Can you work these out from the model? Positions are in its coordinate system, mm. Face numbers are marked on the shaded views. A direction names the side the tool comes from. Round coordinates to 2 decimals unless told otherwise and drop trailing zeros. Write each loop counter-clockwise with the first axis right and the second up, starting at its lowest first coordinate (ties: lowest second). Pieces come first, ordered by that corner, then holes.
Q1. Please list where these lines run through material, in increasing order: line 1 along X through (y, z) = (-50, -14.5); line 2 along X through (y, z) = (-43, -4.5); line 3 along Z through (x, y) = (-13.5, -34).
Q2. We'd pull the mould along Z, two halves only. Please class the marked faces 6, 7 and 8: +Z half, -Z half, draft (parallel to the pull), parting line (faces both ways), or undercut.
Q3. If we section it at B-B (z = 0): Please give me the cut outline in (x, y), plus the area to 3 significant figures.
Q4. For the marked faces 1, 2, 3, 4 and 5, which set-ups out of +Z, -Z, +X, -X, +Y, -Y let a thin tool reach every point of the face, with its end or its side?
Q5. If we section it at A-A (y = -25.5): Please give me the cut outline in (x, z), plus the area to 3 significant figures.
Q6. If we section it at C-C (y = -11): Please give me the cut outline in (x, z), plus the area to 3 significant figures.
Q7. I'm going to push flat-ended pins straight in: pin 1 Ø21 at (x, z) = (-61, 31) entering from -Y; pin 2 Ø8 at (y, z) = (-27, 13.5) entering from -X; pin 3 Ø21 at (x, y) = (-61.5, -27.5) entering from +Z; pin 4 Ø3 at (x, z) = (21, -3.5) entering from +Y. Where does each tip first touch, or does it pass through?
Q8. If we section it at D-D (x = -25): Please give me the cut outline in (y, z).
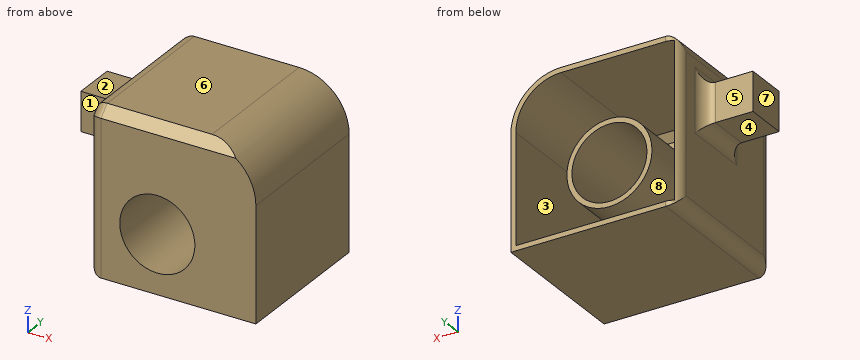
from build123d import *

# Parameters (mm, degrees)
F0_W          = 84.9268175662
F0_H          = 83.4368709475
F1_DEPTH      = 76.2
F2_SIZE       = 5.08
F3_R          = 25.4
F5_D          = 38.1
F8_T          = -2.54
F9_W          = 21.4254707098
F9_H          = 19.7638887912
F10_DEPTH     = 25.4
F11_T1_DEPTH  = 19.7638887912
F11_T3_DEPTH  = 21.4254707098
F11_T9_DEPTH  = 35.6388887912
F11_T13_DEPTH = 37.3004707098
F11_T20_DEPTH = 35.6388887912
F11_T24_DEPTH = 37.3004707098
F11_T31_DEPTH = 37.3004707098
F11_T35_DEPTH = 35.6388887912
F11_T42_DEPTH = 35.6388887912
F11_T46_DEPTH = 37.3004707098
F11_T49_DEPTH = 102.87
F11_T51_DEPTH = 38.9342048969
F11_T53_DEPTH = 115.1868709475
F11_T55_DEPTH = 110.1068709475
F11_T57_DEPTH = 107.95


# Not quite as in the source:
# - a fillet or chamfer that OpenCascade refuses, or shapes differently, is made with other operations: its cross-section is extruded or revolved along the edge and cut away or added


with BuildPart() as f1:
    # F0 (on Front) → F1 (new body)
    with BuildSketch(Plane.XZ):
        with Locations((-3.4268703312, 12.0685463771)):
            Rectangle(F0_W, F0_H)
    extrude(amount=F1_DEPTH)

    # F2
    f2_edges = [f1.edges().sort_by_distance(p)[0] for p in [
        (-3.42687, -76.2, 53.786982),
    ]]
    chamfer(f2_edges, length=F2_SIZE)

    # F3
    f3_edges = [f1.edges().sort_by_distance(p)[0] for p in [
        (39.036538, -35.56, 53.786982),
    ]]
    fillet(f3_edges, radius=F3_R)

    # F5 (through all)
    with Locations(Plane.XZ.offset(76.2)):
        with Locations((-10.9889917076, 0)):
            Hole(F5_D / 2)

    # F8
    f8_openings = [f1.faces().sort_by_distance(p)[0] for p in [
        (-16.12687, 0, 52.596424),
    ]]
    offset(amount=F8_T, openings=f8_openings)

    # F9 (on face) → F10 (join)
    with BuildSketch(Plane(origin=(-45.8902791142, 0, 0), x_dir=(0, -1, 0), z_dir=(-1, 0, 0))):
        with Locations((30.8794565499, 27.0300125703)):
            Rectangle(F9_W, F9_H)
    extrude(amount=F10_DEPTH)

    # F11: fillet of radius 6.35 on 9 edges, made by hand

    # F11_s2 → F11_t1 (join)
    with BuildSketch(Plane.XY.offset(17.1480681747)):
        with BuildLine():
            ThreePointArc((-45.8902791142, -13.816721195), (-47.7501510537, -18.3068492555), (-52.2402791142, -20.166721195))
            Line((-52.2402791142, -20.166721195), (-45.8902791142, -20.166721195))
            Line((-45.8902791142, -20.166721195), (-45.8902791142, -13.816721195))
        make_face()
        with BuildLine():
            ThreePointArc((-45.8902791142, -47.9421919048), (-47.7501510537, -43.4520638442), (-52.2402791142, -41.5921919048))
            Line((-52.2402791142, -41.5921919048), (-45.8902791142, -41.5921919048))
            Line((-45.8902791142, -41.5921919048), (-45.8902791142, -47.9421919048))
        make_face()
    extrude(amount=F11_T1_DEPTH)

    # F11_s4 → F11_t3 (join)
    with BuildSketch(Plane.XZ.offset(20.166721195)):
        with BuildLine():
            ThreePointArc((-45.8902791142, 43.2619569659), (-47.7501510537, 38.7718289054), (-52.2402791142, 36.9119569659))
            Line((-52.2402791142, 36.9119569659), (-45.8902791142, 36.9119569659))
            Line((-45.8902791142, 36.9119569659), (-45.8902791142, 43.2619569659))
        make_face()
        with BuildLine():
            ThreePointArc((-45.8902791142, 10.7980681747), (-47.7501510537, 15.2881962353), (-52.2402791142, 17.1480681747))
            Line((-52.2402791142, 17.1480681747), (-45.8902791142, 17.1480681747))
            Line((-45.8902791142, 17.1480681747), (-45.8902791142, 10.7980681747))
        make_face()
    extrude(amount=F11_T3_DEPTH)


with BuildPart() as f11_tool7:
    # F11_s8 → F11_t9 (new body)
    with BuildSketch(Plane.XY.offset(52.7869569659)):
        with BuildLine():
            ThreePointArc((-45.8902791142, -13.816721195), (-47.7501510537, -18.3068492555), (-52.2402791142, -20.166721195))
            Line((-52.2402791142, -20.166721195), (-45.8902791142, -20.166721195))
            Line((-45.8902791142, -20.166721195), (-45.8902791142, -13.816721195))
        make_face()
    extrude(amount=-F11_T9_DEPTH)

    split(bisect_by=Plane.XY.offset(36.9119569659), keep=Keep.TOP)


with BuildPart() as f11_tool11:
    # F11_s12 → F11_t13 (new body)
    with BuildSketch(Plane.XZ.offset(41.5921919048)):
        with BuildLine():
            ThreePointArc((-45.8902791142, 43.2619569659), (-47.7501510537, 38.7718289054), (-52.2402791142, 36.9119569659))
            Line((-52.2402791142, 36.9119569659), (-45.8902791142, 36.9119569659))
            Line((-45.8902791142, 36.9119569659), (-45.8902791142, 43.2619569659))
        make_face()
    extrude(amount=-F11_T13_DEPTH)

    split(bisect_by=Plane.XZ.offset(20.166721195), keep=Keep.BOTTOM)


with BuildPart() as f11_tool7_1:
    add(f11_tool7.part)

    # F11_t15: intersect F11_tool11
    add(f11_tool11.part, mode=Mode.INTERSECT)


with BuildPart() as f1_1:
    add(f1.part)

    # F11_t5: union F11_tool7
    add(f11_tool7_1.part)


with BuildPart() as f11_tool18:
    # F11_s19 → F11_t20 (new body)
    with BuildSketch(Plane.XY.offset(36.9119569659)):
        with BuildLine():
            ThreePointArc((-45.8902791142, -13.816721195), (-47.7501510537, -18.3068492555), (-52.2402791142, -20.166721195))
            Line((-52.2402791142, -20.166721195), (-45.8902791142, -20.166721195))
            Line((-45.8902791142, -20.166721195), (-45.8902791142, -13.816721195))
        make_face()
    extrude(amount=-F11_T20_DEPTH)

    split(bisect_by=Plane.XY.offset(17.1480681747), keep=Keep.BOTTOM)


with BuildPart() as f11_tool22:
    # F11_s23 → F11_t24 (new body)
    with BuildSketch(Plane.XZ.offset(4.291721195)):
        with BuildLine():
            ThreePointArc((-45.8902791142, 10.7980681747), (-47.7501510537, 15.2881962353), (-52.2402791142, 17.1480681747))
            Line((-52.2402791142, 17.1480681747), (-45.8902791142, 17.1480681747))
            Line((-45.8902791142, 17.1480681747), (-45.8902791142, 10.7980681747))
        make_face()
    extrude(amount=F11_T24_DEPTH)

    split(bisect_by=Plane.XZ.offset(20.166721195), keep=Keep.BOTTOM)


with BuildPart() as f11_tool18_1:
    add(f11_tool18.part)

    # F11_t26: intersect F11_tool22
    add(f11_tool22.part, mode=Mode.INTERSECT)


with BuildPart() as f1_2:
    add(f1_1.part)

    # F11_t16: union F11_tool18
    add(f11_tool18_1.part)


with BuildPart() as f11_tool29:
    # F11_s30 → F11_t31 (new body)
    with BuildSketch(Plane.XZ.offset(57.4671919048)):
        with BuildLine():
            ThreePointArc((-45.8902791142, 43.2619569659), (-47.7501510537, 38.7718289054), (-52.2402791142, 36.9119569659))
            Line((-52.2402791142, 36.9119569659), (-45.8902791142, 36.9119569659))
            Line((-45.8902791142, 36.9119569659), (-45.8902791142, 43.2619569659))
        make_face()
    extrude(amount=-F11_T31_DEPTH)

    split(bisect_by=Plane.XZ.offset(41.5921919048), keep=Keep.TOP)


with BuildPart() as f11_tool33:
    # F11_s34 → F11_t35 (new body)
    with BuildSketch(Plane.XY.offset(17.1480681747)):
        with BuildLine():
            ThreePointArc((-45.8902791142, -47.9421919048), (-47.7501510537, -43.4520638442), (-52.2402791142, -41.5921919048))
            Line((-52.2402791142, -41.5921919048), (-45.8902791142, -41.5921919048))
            Line((-45.8902791142, -41.5921919048), (-45.8902791142, -47.9421919048))
        make_face()
    extrude(amount=F11_T35_DEPTH)

    split(bisect_by=Plane.XY.offset(36.9119569659), keep=Keep.TOP)


with BuildPart() as f11_tool29_1:
    add(f11_tool29.part)

    # F11_t37: intersect F11_tool33
    add(f11_tool33.part, mode=Mode.INTERSECT)


with BuildPart() as f1_3:
    add(f1_2.part)

    # F11_t27: union F11_tool29
    add(f11_tool29_1.part)


with BuildPart() as f11_tool40:
    # F11_s41 → F11_t42 (new body)
    with BuildSketch(Plane.XY.offset(1.2730681747)):
        with BuildLine():
            ThreePointArc((-45.8902791142, -47.9421919048), (-47.7501510537, -43.4520638442), (-52.2402791142, -41.5921919048))
            Line((-52.2402791142, -41.5921919048), (-45.8902791142, -41.5921919048))
            Line((-45.8902791142, -41.5921919048), (-45.8902791142, -47.9421919048))
        make_face()
    extrude(amount=F11_T42_DEPTH)

    split(bisect_by=Plane.XY.offset(17.1480681747), keep=Keep.BOTTOM)


with BuildPart() as f11_tool44:
    # F11_s45 → F11_t46 (new body)
    with BuildSketch(Plane.XZ.offset(20.166721195)):
        with BuildLine():
            ThreePointArc((-45.8902791142, 10.7980681747), (-47.7501510537, 15.2881962353), (-52.2402791142, 17.1480681747))
            Line((-52.2402791142, 17.1480681747), (-45.8902791142, 17.1480681747))
            Line((-45.8902791142, 17.1480681747), (-45.8902791142, 10.7980681747))
        make_face()
    extrude(amount=F11_T46_DEPTH)

    split(bisect_by=Plane.XZ.offset(41.5921919048), keep=Keep.TOP)


with BuildPart() as f11_tool40_1:
    add(f11_tool40.part)

    # F11_t48: intersect F11_tool44
    add(f11_tool44.part, mode=Mode.INTERSECT)


with BuildPart() as f1_4:
    add(f1_3.part)

    # F11_t38: union F11_tool40
    add(f11_tool40_1.part)

    # F11_s50 → F11_t49 (cut)
    with BuildSketch(Plane.XZ.offset(-15.875)):
        with BuildLine():
            ThreePointArc((-39.5402791142, 53.7869818509), (-44.0304071748, 51.9271099114), (-45.8902791142, 47.4369818509))
            Line((-45.8902791142, 47.4369818509), (-45.8902791142, 53.7869818509))
            Line((-45.8902791142, 53.7869818509), (-39.5402791142, 53.7869818509))
        make_face()
    extrude(amount=F11_T49_DEPTH, mode=Mode.SUBTRACT)

    # F11_s52 → F11_t51 (cut)
    with BuildSketch(Plane(origin=(0, 2.5588110768, 2.5588110768), x_dir=(1, 0, 0), z_dir=(0, -0.7071067812, -0.7071067812))):
        with BuildLine():
            ThreePointArc((-45.8902791142, 81.9725738843), (-44.0304071748, 86.4627019448), (-39.5402791142, 88.3225738843))
            Line((-39.5402791142, 88.3225738843), (-45.8902791142, 88.3225738843))
            Line((-45.8902791142, 88.3225738843), (-45.8902791142, 81.9725738843))
        make_face()
    extrude(amount=F11_T51_DEPTH, mode=Mode.SUBTRACT)

    # F11_s54 → F11_t53 (cut)
    with BuildSketch(Plane.XY.offset(-45.5248890966)):
        with BuildLine():
            ThreePointArc((-39.5402791142, 0), (-44.0304071748, -1.8598719395), (-45.8902791142, -6.35))
            Line((-45.8902791142, -6.35), (-45.8902791142, 0))
            Line((-45.8902791142, 0), (-39.5402791142, 0))
        make_face()
    extrude(amount=F11_T53_DEPTH, mode=Mode.SUBTRACT)

    # F11_s56 → F11_t55 (cut)
    with BuildSketch(Plane.XY.offset(-45.5248890966)):
        with BuildLine():
            ThreePointArc((-39.5402791142, -76.2), (-44.0304071748, -74.3401280605), (-45.8902791142, -69.85))
            Line((-45.8902791142, -69.85), (-45.8902791142, -76.2))
            Line((-45.8902791142, -76.2), (-39.5402791142, -76.2))
        make_face()
    extrude(amount=F11_T55_DEPTH, mode=Mode.SUBTRACT)

    # F11_s58 → F11_t57 (cut)
    with BuildSketch(Plane.XZ.offset(-15.875)):
        with BuildLine():
            ThreePointArc((-39.5402791142, -29.6498890966), (-44.0304071748, -27.7900171572), (-45.8902791142, -23.2998890966))
            Line((-45.8902791142, -23.2998890966), (-45.8902791142, -29.6498890966))
            Line((-45.8902791142, -29.6498890966), (-39.5402791142, -29.6498890966))
        make_face()
    extrude(amount=F11_T57_DEPTH, mode=Mode.SUBTRACT)


solid = f1_4.part
A:
1. line 1: x = -45.89 to -43.35, -26.99 to -23.34, 1.37 to 5.01, 36.5 to 39.04
1. line 2: x = -45.89 to -43.35, -32.1 to -29.5, 7.52 to 10.13, 36.5 to 39.04
1. line 3: z = -29.65 to -27.11, -21.44 to -18.88, 18.88 to 21.44, 51.25 to 53.79
2. face 6: +Z half
2. face 7: draft
2. face 8: undercut
3. outline: (-45.89, -69.85) arc R6.35 ccw to (-39.54, -76.2) - (-30.04, -76.2) - (-30.04, 0) - (-32.58, 0) - (-32.58, -73.66) - (-43.35, -73.66) - (-43.35, -1.27) arc R6.35 ccw to (-45.89, -6.35) - close; (8.06, -76.2) - (39.04, -76.2) - (39.04, 0) - (36.5, 0) - (36.5, -73.66) - (10.6, -73.66) - (10.6, 0) - (8.06, 0) - close
3. area: 852 mm2
4. face 1: +Z, -Z, -X, -Y
4. face 2: +Z, -X, +Y, -Y
4. face 3: +Y
4. face 4: -Z, -X, +Y, -Y
4. face 5: +Z, -Z, -X, +Y
5. outline: (-71.29, 17.15) - (-52.24, 17.15) arc R6.35 cw to (-45.89, 10.8) - (-45.89, -23.3) arc R6.35 ccw to (-39.54, -29.65) - (39.04, -29.65) - (39.04, 28.39) arc R25.4 ccw to (13.64, 53.79) - (-39.54, 53.79) arc R6.35 ccw to (-45.89, 47.44) - (-45.89, 43.26) arc R6.35 cw to (-52.24, 36.91) - (-71.29, 36.91) - close; circle Ø43.18 at (-10.99, 0); hole (-43.35, -27.11) - (36.5, -27.11) - (36.5, 28.39) arc R22.86 ccw to (13.64, 51.25) - (-43.35, 51.25) - close; hole circle Ø38.1 at (-10.99, 0)
5. area: 1,630 mm2
6. outline: (-45.89, -23.3) arc R6.35 ccw to (-39.54, -29.65) - (39.04, -29.65) - (39.04, 28.39) arc R25.4 ccw to (13.64, 53.79) - (-39.54, 53.79) arc R6.35 ccw to (-45.89, 47.44) - close; circle Ø43.18 at (-10.99, 0); hole (-43.35, -27.11) - (36.5, -27.11) - (36.5, 28.39) arc R22.86 ccw to (13.64, 51.25) - (-43.35, 51.25) - close; hole circle Ø38.1 at (-10.99, 0)
6. area: 1,110 mm2
7. pin 1: stops at y = -41.84
7. pin 2: stops at x = -71.29
7. pin 3: stops at z = 37.03
7. pin 4: stops at y = -73.66
8. outline: (-76.2, -29.65) - (0, -29.65) - (0, -27.11) - (-73.66, -27.11) - (-73.66, -16.43) - (0, -16.43) - (0, -12.91) - (-76.2, -12.91) - close; (-76.2, 12.91) - (0, 12.91) - (0, 16.43) - (-73.66, 16.43) - (-73.66, 47.65) - (-70.07, 51.25) - (0, 51.25) - (0, 53.79) - (-71.12, 53.79) - (-76.2, 48.71) - close
